Build history of the part. All positions in model axes, mm. A direction names the side the tool comes from. Round coordinates to 2 decimals unless told otherwise and drop trailing zeros. Write each loop counter-clockwise with the first axis right and the second up, starting at its lowest first coordinate (ties: lowest second). Pieces come first, ordered by that corner, then holes. Notation, with made-up numbers: (19, 85.25) - (59, 85.25) arc R23 cw to (59, 106.25) - close; hole circle Ø5 at (-30, 18.5). An arc over 180 degrees is marked (long way). Write each question's results on one line, items separated by ' | '.
from build123d import *

# Parameters (mm, degrees)
F1_DEPTH = 21.844
F2_DEPTH = 95.25
F3_R     = 16.86574
F4_DEPTH = 63.5


with BuildPart() as f1:
    # F0 (on Front) → F1 (new body)
    with BuildSketch(Plane.XZ):
        Polygon((62.899669, -56.346651), (0, 56.346651), (-62.899669, 56.346651), (-62.899669, 40.344652), (-9.394319, 40.344652), (44.573848, -56.346651), align=None)
        Polygon((-9.394319, 40.344652), (-62.899669, 40.344652), (-62.899669, -56.346651), (44.573848, -56.346651), align=None)
    extrude(amount=-F1_DEPTH)

    # F0 (on Front) → F2 (join)
    with BuildSketch(Plane.XZ):
        Polygon((-9.394319, 40.344652), (-62.899669, 40.344652), (-62.899669, -56.346651), (44.573848, -56.346651), align=None)
    extrude(amount=F2_DEPTH)

    # F3 (on Right) → F4 (cut, symmetric)
    with BuildSketch(Plane.YZ):
        with Locations((-38.252983, 0)):
            Circle(F3_R)
    extrude(amount=F4_DEPTH, both=True, mode=Mode.SUBTRACT)


solid = f1.part
(1) Drill centre lines: probe 1 along Y at (x, z) = (-44, 0); probe 2 along Y at (x, z) = (15, 29); probe 3 along X at (y, z) = (-72.5, 23.5). Where is each one in solid material? Low to high. Write a range as [from, to].
Worked answers:
probe 1: y = [-95.25, -55.12], [-21.39, 21.84] | probe 2: y = [0, 21.84] | probe 3: x = [-62.9, 0.01]
(2) Two-plate mould, pull along Y, no slides. Class faces 4 (the cylindrical face through (-19.583, -41.909, -16.465)), 5 (the flat face through (-1, -36, -56.347)), 6 (the flat face through (-15, 21.844, 1)), 7 (the flat face through (-22, -95.25, -7)): released by +Y, released by -Y, zero draft, split by the parting line, or undercut.
Worked answers:
face 4: undercut | face 5: zero draft | face 6: released by +Y | face 7: released by -Y
(3) Slice it at A-A, the plane x = -14. Write the cut outline in (y, z), and give its area (3 significant figures).
Worked answers:
outline: (-95.25, -56.35) - (21.84, -56.35) - (21.84, 56.35) - (0, 56.35) - (0, 40.34) - (-95.25, 40.34) - close; hole circle Ø33.73 at (-38.25, 0) | area: 10,800 mm2
(4) Slice it at D-D, the plane z = 14. Write the cut outline in (x, y), and give its area (3 significant figures).
Worked answers:
outline: (-62.9, -95.25) - (5.31, -95.25) - (5.31, -47.66) - (-62.9, -47.66) - close; (-62.9, -28.85) - (5.31, -28.85) - (5.31, 0) - (23.64, 0) - (23.64, 21.84) - (-62.9, 21.84) - close | area: 7,100 mm2
(5) Tool access for faces 1 (the flat face through (-36, -47, 40.345)), 2 (the flat face through (-62.9, -23, -12)), 3 (the flat face through (9, 0, 13)): list every direction of +Z, -Z, +X, -X, +Y, -Y with a clear straight run to the whole face (end or side of a thin tool).
Worked answers:
face 1: +Z, +X, -X, -Y | face 2: +Z, -Z, -X, +Y, -Y | face 3: +Z, +X, -Y
(6) Slice it at B-B, the plane y = -34.5. Write the cut outline in (x, z), and give its area (3 significant figures).
Worked answers:
outline: (-62.9, -56.35) - (44.57, -56.35) - (22.3, -16.44) - (-62.9, -16.44) - close; (-62.9, 16.44) - (3.95, 16.44) - (-9.39, 40.34) - (-62.9, 40.34) - close | area: 5,280 mm2
(7) Flat gauge pins, fed straight in: pin 1 Ø3 at (y, z) = (-11.5, -7) entering from +X; pin 2 Ø3 at (x, y) = (15.5, -28) entering from +Z; pin 3 Ø1 at (y, z) = (0.5, 39) entering from +X. Where does each tip first touch, or does it go through?
Worked answers:
pin 1: stops at x = 17.87 | pin 2: stops at z = -12.1 | pin 3: stops at x = 9.96
(8) Slice it at C-C, the plane z = 0. Write the cut outline in (x, y), and give its area (3 significant figures).
Worked answers:
outline: (-62.9, -95.25) - (13.12, -95.25) - (13.12, -55.12) - (-62.9, -55.12) - close; (-62.9, -21.39) - (13.12, -21.39) - (13.12, 0) - (31.45, 0) - (31.45, 21.84) - (-62.9, 21.84) - close | area: 6,740 mm2
